The listing builds one solid part. Answer for the finished solid, in the listing's coordinates (mm). A direction names the side the tool comes from. Round coordinates to 2 decimals unless told otherwise and drop trailing zeros. Loops run counter-clockwise (first coordinate to the right, second up) from the corner with the lowest first, then second, coordinate; pieces in that order, holes last. Notation, with made-up numbers: (-16.5, 79) - (5.5, 79) arc R15 ccw to (5.5, 102) - close; hole circle Ø4 at (44, -30). An arc over 180 degrees is marked (long way). One line per item, written item: value.
```python
from build123d import *

# Parameters (mm, degrees)
SKETCH1_R           = 1.7
SKETCH1_R_2         = 1.5875
BOSS_EXTRUDE1_DEPTH = 2
SKETCH2_W           = 38.1
SKETCH2_H           = 2
BOSS_EXTRUDE2_DEPTH = 38.1
SKETCH3_R           = 3.175
CUT_EXTRUDE1_DEPTH  = 63.903065307


with BuildPart() as part:
    # Sketch1 → Boss-Extrude1 (new body)
    with BuildSketch(Plane(origin=(0, 0, 0), x_dir=(1, 0, 0), z_dir=(0, 1, 0))):
        Polygon((-25.4, 15.875), (12.7, 15.875), (12.7, 25.4), (25.4, 25.4), (25.4, -25.4), (12.7, -25.4), (12.7, -15.875), (-25.4, -15.875), align=None)
        with Locations(Location((19.05, 20.6375, 0), (0, 0, 270))):
            Circle(SKETCH1_R, mode=Mode.SUBTRACT)
        with Locations(Location((19.05, -20.6375, 0), (0, 0, 270))):
            Circle(SKETCH1_R, mode=Mode.SUBTRACT)
        with Locations(Location((0, 6.35, 0), (0, 0, 270))):
            Circle(SKETCH1_R_2, mode=Mode.SUBTRACT)
        with Locations(Location((0, -6.35, 0), (0, 0, 270))):
            Circle(SKETCH1_R_2, mode=Mode.SUBTRACT)
    extrude(amount=BOSS_EXTRUDE1_DEPTH)

    # Sketch2 → Boss-Extrude2 (add)
    with BuildSketch(Plane(origin=(0, 2, 0), x_dir=(1, 0, 0), z_dir=(0, 1, 0))):
        with Locations((-6.35, 14.875)):
            Rectangle(SKETCH2_W, SKETCH2_H)
        with Locations((-6.35, -14.875)):
            Rectangle(SKETCH2_W, SKETCH2_H)
    extrude(amount=BOSS_EXTRUDE2_DEPTH)

    # Sketch3 → Cut-Extrude1 (cut, through all)
    with BuildSketch(Plane.XY.offset(15.875)):
        with Locations((-5.6, 30.16795818)):
            Circle(SKETCH3_R)
    extrude(amount=-CUT_EXTRUDE1_DEPTH, mode=Mode.SUBTRACT)


solid = part.part
```
1) Each of these flat-tipped pins is pushed along its axis until it touches: pin 1 Ø1 at (x, y) = (11, 14) entering from +Z (3 decimals); pin 2 Ø10 at (x, y) = (-16.5, 7) entering from -Z (3 decimals); pin 3 Ø3 at (x, z) = (0, -6.35) entering from +Y; pin 4 Ø0.6 at (y, z) = (1, 18.5) entering from -X. Where does it stop, or does it pass through?
Final values:
pin 1: z = 15.875
pin 2: z = -15.875
pin 3: through
pin 4: x = 12.7
2) For a pull along X with two mould halves and no side action, classify faces 1 (the cylindrical face through (19.56, 0.99, 22.26)), 2 (the flat face through (-25.4, 17, 14.2)), 3 (the flat face through (-7, 40.1, -15)) as released by +X, released by -X, zero draft, split by the parting line, or undercut.
Final values:
face 1: undercut
face 2: released by -X
face 3: zero draft
3) A cutting plane is placed at D-D on x = -21. Give the vertices of the cut face in (y, z) (3 decimals), and give its area (3 significant figures).
Final values:
outline: (0, -15.875) - (40.1, -15.875) - (40.1, -13.875) - (2, -13.875) - (2, 13.875) - (40.1, 13.875) - (40.1, 15.875) - (0, 15.875) - close
area: 216 mm2
4) A cutting plane is placed at C-C on z = 6.35. Give the vertices of the cut face in (x, y), and give its area (4 significant figures).
Final values:
outline: (-25.4, 0) - (-1.59, 0) - (-1.59, 2) - (-25.4, 2) - close; (1.59, 0) - (25.4, 0) - (25.4, 2) - (1.59, 2) - close
area: 95.25 mm2
5) Consider L1, parallel to Z at x = -12.5, y = 28 (3 decimals); L2, parallel to Z at x = 19, y = 1; L3, parallel to Y at x = -5.6, z = 15.45. Determine where each line is inside the solid, lowest interval first.
Final values:
L1: -15.875 to -13.875, 13.875 to 15.875
L2: -25.4 to -22.34, -18.94 to 18.94, 22.34 to 25.4
L3: 0 to 26.99, 33.34 to 40.1
6) A cutting plane is placed at A-A on y = 10. Give the vertices of the cut face in (x, z) (3 decimals), and give its area (3 significant figures).
Final values:
outline: (-25.4, -15.875) - (12.7, -15.875) - (12.7, -13.875) - (-25.4, -13.875) - close; (-25.4, 13.875) - (12.7, 13.875) - (12.7, 15.875) - (-25.4, 15.875) - close
area: 152 mm2
7) A cutting plane is placed at B-B on x = 0. Give the vertices of the cut face in (y, z) (1 decimal), and give its area (3 significant figures).
Final values:
outline: (0, -15.9) - (40.1, -15.9) - (40.1, -13.9) - (2, -13.9) - (2, -7.9) - (0, -7.9) - close; (0, -4.8) - (2, -4.8) - (2, 4.8) - (0, 4.8) - close; (0, 7.9) - (2, 7.9) - (2, 13.9) - (40.1, 13.9) - (40.1, 15.9) - (0, 15.9) - close
area: 203 mm2
8) For faces 4 (the flat face through (-7, 21, -13.875)), 5 (the flat face through (12.7, 1, 21)), 6 (the flat face through (12.7, 1, -21)), determine the directions among +Z, -Z, +X, -X, +Y, -Y from which every point of the face is accessible in a straight line to the end or side of a thin tool.
Final values:
face 4: +X, -X, +Y
face 5: +Z, -X, +Y, -Y
face 6: -Z, -X, +Y, -Y
